Read the model definition and answer for the solid it produces. Units are mm, in the model's axes. Face numbers are marked on the shaded views. A direction names the side the tool comes from. Coordinates: 2 decimals unless noted, no trailing zeros. Order: outer loops, then holes, each group sorted by start corner. A loop starts at its lowest first (then second) coordinate and runs counter-clockwise, first axis right, second up. Notation, with made-up numbers: (-18, 19.5) -> (41, 19.5) arc R32 cw to (41, 49.5) -> close; hole circle Ø5 at (66, 45.25). An arc over 180 degrees is marked (long way). Use CSV: the item, a comma, the result in double quotes.
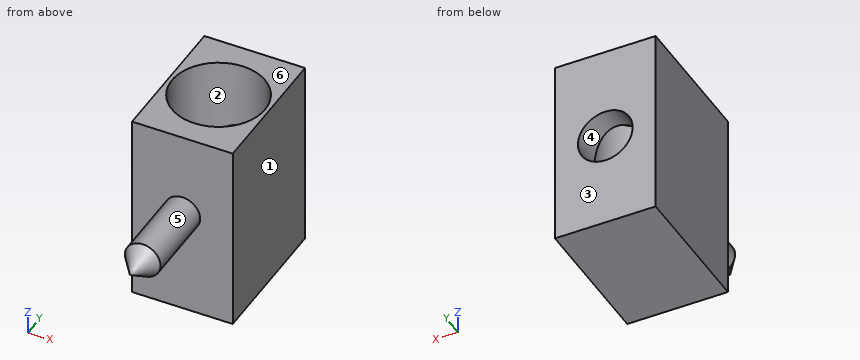
```python
from build123d import *

# Parameters (mm, degrees)
SKETCH1_W           = 3.68
SKETCH1_H           = 7
BOSS_EXTRUDE1_DEPTH = 5.1
SKETCH2_R           = 1.7
CUT_EXTRUDE1_DEPTH  = 6.5
SKETCH3_R           = 0.65
BOSS_EXTRUDE2_DEPTH = 2.8
CUT_EXTRUDE2_REACH  = 9.9
SKETCH4_R           = 1


with BuildPart() as part:
    # Sketch1 → Boss-Extrude1 (new body)
    with BuildSketch(Plane(origin=(0, 0, 0), x_dir=(1, 0, 0), z_dir=(0, 1, 0))):
        with Locations((-1.84, -3.5)):
            Rectangle(SKETCH1_W, SKETCH1_H)
    extrude(amount=BOSS_EXTRUDE1_DEPTH)

    # Sketch2 → Cut-Extrude1 (cut)
    with BuildSketch(Plane.XY.offset(7)):
        with Locations((-1.84, 2.55)):
            Circle(SKETCH2_R)
    extrude(amount=-CUT_EXTRUDE1_DEPTH, mode=Mode.SUBTRACT)

    # Sketch3 → Boss-Extrude2 (add)
    with BuildSketch(Plane.XZ):
        with Locations((-1.84, 3.9)):
            Circle(SKETCH3_R)
    extrude(amount=BOSS_EXTRUDE2_DEPTH)

    # Sketch4 → Cut-Extrude2 (cut, up to next)
    with BuildSketch(Plane(origin=(0, 5.1, 0), x_dir=(1, 0, 0), z_dir=(0, 1, 0)), mode=Mode.PRIVATE) as cut_extrude2_sk1:
        with Locations((-1.84, -3.55)):
            Circle(SKETCH4_R)
    cut_extrude2_tool1 = extrude(cut_extrude2_sk1.sketch, amount=-CUT_EXTRUDE2_REACH, mode=Mode.PRIVATE) & part.part
    add(cut_extrude2_tool1.solids().sort_by_distance((-1.84, 5.1, 3.55))[0], mode=Mode.SUBTRACT)

    # Sketch7 → Revolve2 (revolve)
    with BuildSketch(Plane(origin=(-1.84, 0, 0), x_dir=(0, 0, -1), z_dir=(1, 0, 0))):
        Polygon((-3.9, -2.8), (-3.9, -3.7), (-4.55, -2.8), align=None)
    revolve(axis=Axis((-1.84, -2.8, 3.9), (0, -1, 0)))


solid = part.part
```
Item 1: Find section D-D, the plane y = -0.25. Give the vertices of the cut face in (x, z), then the cut area to 3 significant figures.
Return value:
outline,"circle Ø1.3 at (-1.84, 3.9)"
area,"1.33 mm^2"
Item 2: The mould has two halves that part along Y. Classify the marked faces 1, 2 and 3: +Y half, -Y half, draft (parallel to the pull), parting line (faces both ways), or undercut.
Return value:
face 1,"draft"
face 2,"undercut"
face 3,"+Y half"
Item 3: Find section C-C, the plane x = -0.4. Give the vertices of the cut face in (y, z), then the cut area to 3 significant figures.
Return value:
outline,"(0, 0) -> (5.1, 0) -> (5.1, 7) -> (3.45, 7) -> (3.45, 0.5) -> (1.65, 0.5) -> (1.65, 7) -> (0, 7) -> close"
area,"24.0 mm^2"
Item 4: Each of these flat-tipped pins is pushed along its axis until it touches: P1, Ø1, axis at x = -1.5, y = 2.5, coming from the +Z side; P2, Ø1.6, axis at x = -1.84, z = 3.55, coming from the +Y side. Where does it stop, or does it pass through?
Return value:
P1,"stops at z = 0.5"
P2,"stops at y = 1.05"
Item 5: Find section A-A, the plane y = 1.75. Give the vertices of the cut face in (x, z).
Return value:
outline,"(-3.68, 0) -> (0, 0) -> (0, 7) -> (-0.34, 7) -> (-0.34, 0.5) -> (-3.34, 0.5) -> (-3.34, 7) -> (-3.68, 7) -> close"
Item 6: Find section B-B, the plane z = 4.75. Give the vertices of the cut face in (x, y), then the cut area to 3 significant figures.
Return value:
outline,"(-3.68, 0) -> (0, 0) -> (0, 5.1) -> (-3.68, 5.1) -> close; hole circle Ø3.4 at (-1.84, 2.55)"
area,"9.69 mm^2"
Item 7: Straight lines are drawn through the part: line 1 along X through (y, z) = (4.95, 3.55); line 2 along Z through (x, y) = (-1.84, 4.8); line 3 along Y through (x, z) = (-1.84, 4.75). For each, find the intervals that lie inside material, in ascending order.
Return value:
line 1,"x = -3.68 to -2.84, -0.84 to 0"
line 2,"z = 0 to 2.55, 4.55 to 7"
line 3,"y = 0 to 0.85, 4.25 to 5.1"
Item 8: A tool of negligible diameter and unlimited length cuts with its end or side. For the marked faces 4, 5 and 6, from which of +Z, -Z, +X, -X, +Y, -Y can it reach the whole face along a straight path? Write none if from no direction.
Return value:
face 4,"+Y"
face 5,"-Y"
face 6,"+Z, +X, -X, +Y, -Y"
